Check sheet for the drawn part. Datum: minimum x, y, z corner. Units: mm. A direction names the side the tool comes from. Coordinates: 2 decimals unless noted, no trailing zeros. Order: outer loops, then holes, each group sorted by start corner. A loop starts at its lowest first (then second) coordinate and runs counter-clockwise, first axis right, second up.
1. Gauge pin test, flat ends, axial feed: pin 1 Ø2.5 at (x, z) = (80.5, 29.5) entering from +Y; pin 2 Ø0.9 at (y, z) = (2, 44.5) entering from +X; pin 3 Ø3 at (x, y) = (71.5, 6) entering from +Z. Record the tip position at first contact, or that the pin passes through.
2. Cross-section at A-A (x = 53). Enter the section's corners in (y, z).
3. Thickness scan on line 1 (X direction, y = 3.6, z = 4.25); line 2 (Z direction, x = 82, y = 3.8); line 3 (Z direction, x = 54.5, y = 6.75). Record the ranges inside material, lowest first.
4. Cross-section at C-C (z = 14). Enter the section's corners in (x, y), then the cut area to 3 significant figures.
5. Cross-section at B-B (z = 40.5). Enter the section's corners in (x, y).
6. Cross-section at D-D (x = 76). Enter the section's corners in (y, z), then the cut area to 3 significant figures.
7. Set-up check for the marked faces 1 and 2: record each of +Z, -Z, +X, -X, +Y, -Y from which the full face is reachable in a straight line by a thin tool's end or side.
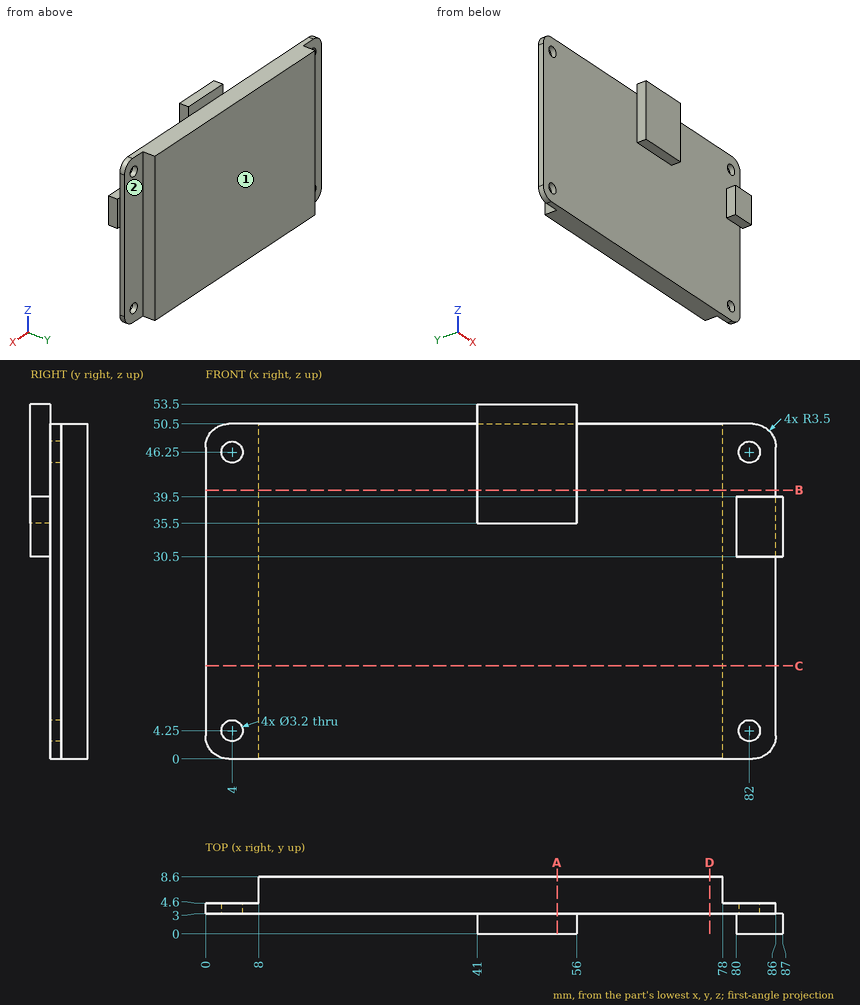
Data:
1. pin 1: stops at y = 4.6
1. pin 2: stops at x = 56
1. pin 3: stops at z = 50.5
2. outline: (0, 35.5) - (3, 35.5) - (3, 0) - (8.6, 0) - (8.6, 50.5) - (3, 50.5) - (3, 53.5) - (0, 53.5) - close
3. line 1: x = 0 to 2.4, 5.6 to 80.4, 83.6 to 86
3. line 2: z = 0 to 2.65, 5.85 to 44.65, 47.85 to 50.5
3. line 3: z = 0 to 50.5
4. outline: (0, 3) - (86, 3) - (86, 4.6) - (78, 4.6) - (78, 8.6) - (8, 8.6) - (8, 4.6) - (0, 4.6) - close
4. area: 418 mm2
5. outline: (0, 3) - (41, 3) - (41, 0) - (56, 0) - (56, 3) - (86, 3) - (86, 4.6) - (78, 4.6) - (78, 8.6) - (8, 8.6) - (8, 4.6) - (0, 4.6) - close
6. outline: (3, 0) - (8.6, 0) - (8.6, 50.5) - (3, 50.5) - close
6. area: 283 mm2
7. face 1: +Z, -Z, +X, -X, +Y
7. face 2: +Z, -Z, +X, +Y
